Design review of the part built by this model. Coordinates are the model's own, in mm. A direction names the side the tool comes from. Give positions to 0.01 mm unless a question says otherwise; leave off trailing zeros. Write each loop counter-clockwise with the first axis right and the second up, starting at its lowest first coordinate (ties: lowest second). Pieces come first, ordered by that corner, then holes. Notation, with made-up numbers: M 34.5,8 L 73.5,8 A23 cw 73.5,44 Z; hole C -28.5,-29 d8. An arc over 180 degrees is marked long. Use one line per item in the form item = value. Start each with the question number.
from build123d import *

# Parameters (mm, degrees)
F0_R     = 3.75
F0_R_2   = 2.5
F1_DEPTH = 0.8
F3_DEPTH = 6.7


with BuildPart() as f1:
    # F0 (on Top) → F1 (new body)
    with BuildSketch(Plane.XY):
        Circle(F0_R)
        Circle(F0_R_2, mode=Mode.SUBTRACT)
    extrude(amount=F1_DEPTH)

    # F2 (on face) → F3 (join)
    with BuildSketch(Plane(origin=(0, 0, 0), x_dir=(1, 0, 0), z_dir=(0, 0, -1))):
        with BuildLine():
            Line((-2.193171, -1.2), (-3.074085, -1.2))
            ThreePointArc((-3.074085, -1.2), (0, -3.3), (3.074085, -1.2))
            Line((3.074085, -1.2), (2.193171, -1.2))
            ThreePointArc((2.193171, -1.2), (0, -2.5), (-2.193171, -1.2))
        make_face()
        with BuildLine():
            ThreePointArc((3.074085, 1.2), (0, 3.3), (-3.074085, 1.2))
            Line((-3.074085, 1.2), (-2.193171, 1.2))
            ThreePointArc((-2.193171, 1.2), (0, 2.5), (2.193171, 1.2))
            Line((2.193171, 1.2), (3.074085, 1.2))
        make_face()
    extrude(amount=F3_DEPTH)


solid = f1.part
1. To check wall thickness, follow L1, parallel to Y at x = 0, z = 0.2; L2, parallel to Y at x = -1, z = -1.5; L3, parallel to Z at x = 2.25, y = 2.5. State the ranges of each line that lie inside material, in increasing order.
2. Draft analysis for pull direction Y (two halves, no side actions). For faces 4 (the flat face through (0, 3, -6.7)), 5 (the flat face through (-3, 0, 0)), 6 (the cylindrical face through (0.1, -3.3, -3.3)), state which applies: pulls with the +Y half, pulls with the -Y half, needs draft (parallel to the pull), parting line crosses it, or undercut.
3. We need section D-D (y = -3). State the section outline as (x, z) points.
4. We need section B-B (x = 0). State the section outline as (y, z) points.
5. For faces 1 (the cylindrical face through (-0.1, 3.3, -3.3)), 2 (the cylindrical face through (-3.746, 0.165, 0.394)), 3 (the flat face through (2.6, 1.2, -3.3)), list the 3-axis set-ups (+Z, -Z, +X, -X, +Y, -Y) from which the entire face can be reached by the end or side of a thin tool; tool diameter is ignored.
6. We need section C-C (z = -4.5). State the section outline as (x, y) points, and give its area (3 significant figures).
7. Clearance check with flat-ended pins moving along their axes: pin 1 Ø4 at (y, z) = (2, -2.5) entering from +X; pin 2 Ø2 at (y, z) = (-2.5, -0.5) entering from -X; pin 3 Ø1 at (x, z) = (2.5, -4) entering from +Y; pin 4 Ø1 at (y, z) = (0, -5) entering from -X. State where each tip first meets the part, or that it passes through.
8. We need section A-A (y = 0). State the section outline as (x, z) points.
Answer block:
q1.L1 = -3.75 to -2.5, 2.5 to 3.75
q1.L2 = -3.14 to -2.29, 2.29 to 3.14
q1.L3 = 0 to 0.8
q2.face_4 = needs draft
q2.face_5 = undercut
q2.face_6 = pulls with the -Y half
q3.outline = M -2.25,0 L -1.37,0 L -1.37,-6.7 L 1.37,-6.7 L 1.37,0 L 2.25,0 L 2.25,0.8 L -2.25,0.8 Z
q4.outline = M -3.75,0 L -3.3,0 L -3.3,-6.7 L -2.5,-6.7 L -2.5,0.8 L -3.75,0.8 Z; M 2.5,-6.7 L 3.3,-6.7 L 3.3,0 L 3.75,0 L 3.75,0.8 L 2.5,0.8 Z
q5.face_1 = -Z, +Y
q5.face_2 = +Z, -Z
q5.face_3 = -Z, +X, -X
q6.outline = M -3.07,-1.2 A3.3 ccw 3.07,-1.2 L 2.19,-1.2 A2.5 cw -2.19,-1.2 Z; M -3.07,1.2 L -2.19,1.2 A2.5 cw 2.19,1.2 L 3.07,1.2 A3.3 ccw Z
q6.area = 10.6 mm^2
q7.pin_1 = 3.07
q7.pin_2 = -3.38
q7.pin_3 = 2.62
q7.pin_4 = through
q8.outline = M -3.75,0 L -2.5,0 L -2.5,0.8 L -3.75,0.8 Z; M 2.5,0 L 3.75,0 L 3.75,0.8 L 2.5,0.8 Z
